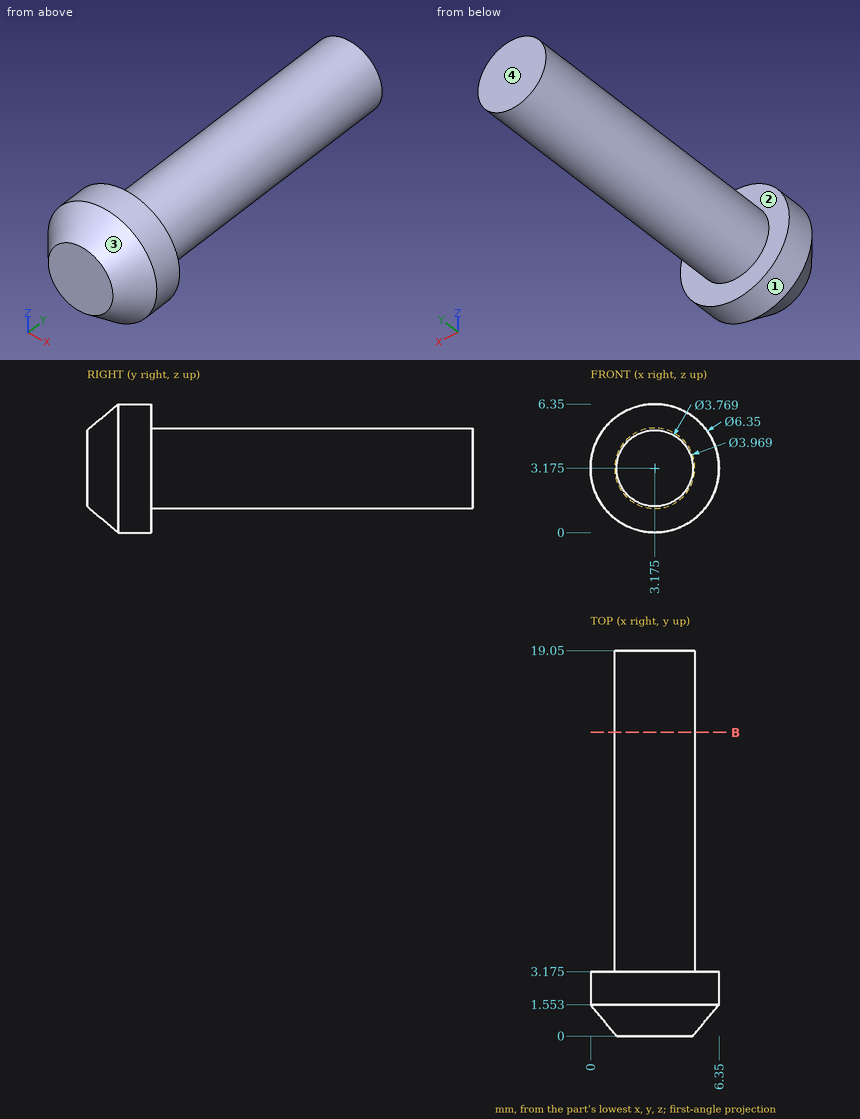
The drawing under review shows one solid part. Ordinate dimensions are in mm from its lowest x, y, z. A direction names the side the tool comes from. Coordinates: 2 decimals unless noted, no trailing zeros. Write each loop counter-clockwise with the first axis right and the second up, starting at its lowest first coordinate (ties: lowest second). Pieces come first, ordered by that corner, then holes. Notation, with made-up numbers: (22, 88) - (50, 88) arc R29 cw to (50, 123) - close; hole circle Ø3 at (86.5, 10.5). An arc over 180 degrees is marked (long way). Answer in a Markdown table with one row per item. Add a question column.
Q1. For P1, Ø1, axis at x = 3.5, y = 13.5, coming from the +Z side; P2, Ø1, axis at x = 2.5, y = 2, coming from the -Z side (1 decimal); P3, Ø2, axis at y = 9, z = 4, coming from the +X side, all flat-tipped, find the tip position at first contact; note any pin that passes through.
Q2. For probe 1 along X at (y, z) = (4, 3.25); probe 2 along Z at (x, y) = (2.25, 15.25); probe 3 along Z at (x, y) = (0.75, 1.75) (1 decimal), list the stretches that pass through material, from the lowest coordinate up.
Q3. Tool access review of the marked faces 1 and 2: name each direction out of +Z, -Z, +X, -X, +Y, -Y from which nothing blocks a thin tool from reaching the whole face with its end or side.
Q4. We need section B-B, the plane y = 15. State the section outline as (x, z) points (1 decimal), and give its area (3 significant figures).
Q5. Draft analysis for pull direction Z (two halves, no side actions). For the marked faces 3 and 4, state which applies: +Z half, -Z half, draft (parallel to the pull), parting line (faces both ways), or undercut.
Answer list:
| question | item | result |
|---|---|---|
| 1 | P1 | stops at z = 5.16 |
| 1 | P2 | stops at z = 0 |
| 1 | P3 | stops at x = 5.16 |
| 2 | probe 1 | x = 1.19 to 5.16 |
| 2 | probe 2 | z = 1.42 to 4.93 |
| 2 | probe 3 | z = 1.1 to 5.2 |
| 3 | face 1 | +Y, -Y |
| 3 | face 2 | +Y |
| 4 | outline | circle Ø4 at (3.2, 3.2) |
| 4 | area | 12.4 mm2 |
| 5 | face 3 | parting line |
| 5 | face 4 | draft |
